The listing builds one solid part. Answer for the finished solid, in the listing's coordinates (mm). Face numbers are marked on the shaded views. Give positions to 0.01 mm unless a question says otherwise; leave off trailing zeros. Write each loop counter-clockwise with the first axis right and the second up, starting at its lowest first coordinate (ties: lowest second). Pieces come first, ordered by that corner, then holes. Notation, with made-up numbers: (-19.5, -1.5) - (34.5, -1.5) arc R25 cw to (34.5, 15.5) - close; hole circle Ø8 at (58.25, -21). An arc over 180 degrees is marked (long way). Use a Markdown table: item, result. Add a question column.
Autodesk Inventor part; units mm, degrees
ref_plane "YZ Plane" through (0, 0, 0) normal (1, 0, 0) x (0, 1, 0)
ref_plane "XZ Plane" through (0, 0, 0) normal (0, 1, 0) x (-1, 0, 0)
ref_plane "XY Plane" through (0, 0, 0) normal (0, 0, 1) x (1, 0, 0)
sketch "Sketch1" plane through (0, 0, 0) normal (0, 1, 0) x (-1, 0, 0)
  line L0 (-4, -15) -> (4, -15)
  line L1 (4, -15) -> (4, 15)
  line L2 (4, 15) -> (-4, 15)
  line L3 (-4, 15) -> (-4, -15)
  line L4 (-4, -15) -> (4, 15) construction
  line L5 (4, -15) -> (-4, 15) construction
  circle A0 centre (0, 0) radius 1.75
  dimension "d0" = 8
  dimension "d1" = 30
  dimension "d2" = 3.5
extrude "Extrusion1" add sketch "Sketch1" along normal blind 5
sketch "Sketch2" plane through (0, 5, 0) normal (0, 1, 0) x (1, 0, 0)
  circle A0 centre (0, 0) radius 1.75
  circle A1 centre (0, 0) radius 2.75 construction
  line L0 (-2.75, 1.5877) -> (0, 3.1754)
  line L1 (0, 3.1754) -> (2.75, 1.5877)
  line L2 (2.75, 1.5877) -> (2.75, -1.5877)
  line L3 (2.75, -1.5877) -> (0, -3.1754)
  line L4 (0, -3.1754) -> (-2.75, -1.5877)
  line L5 (-2.75, -1.5877) -> (-2.75, 1.5877)
  point P0 (-2.75, 0)
  dimension "d5" = 5.5
extrude "Extrusion2" cut sketch "Sketch2" against normal blind 2.4 contours A0 | L0 L1 L2 L3 L4 L5
sketch "Sketch3" plane through (0, 5, 0) normal (0, 1, 0) x (1, 0, 0)
  line L0 (-4, -15) -> (4, -15)
  line L1 (0, -15) -> (0, 15) construction
  line L2 (4, 15) -> (-4, 15)
  point P0 (0, 0)
  point P1 (0, -10)
  point P2 (0, 10)
  dimension "d8" = 5
  dimension "d9" = 5
hole "Hole1" at (0, 5, 10) at (0, 5, -10) direction (0, -1, 0) diameter 3.4 end through all
properties part number "turning clip bottom"
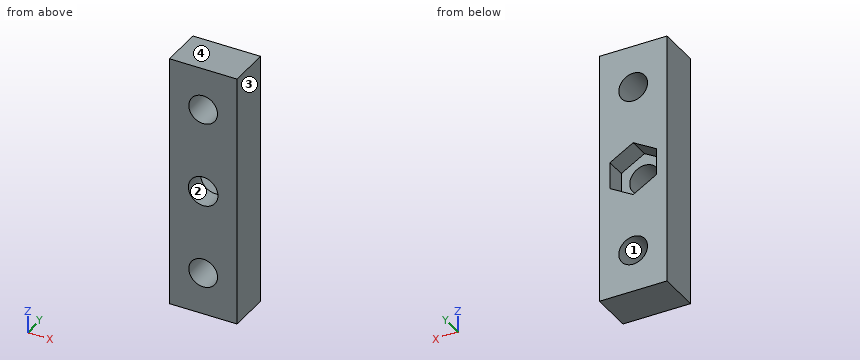
1. Consider L1, parallel to Z at x = 0, y = 1.35; L2, parallel to X at y = 1.7, z = 0; L3, parallel to Z at x = -0.75, y = 0.3. Determine where each line is inside the solid, lowest interval first. Write a range as [from, to].
2. The part is cut by section C-C (x = 0.75). Give the vertices of the cut face in (y, z).
3. Given P1, Ø4.5, axis at x = -0.5, z = 1, coming from the +Y side, flat-ended and moving along its own axis, determine where the tip first touches the part or whether it passes through.
4. The part is cut by section D-D (z = 0). Give the vertices of the cut face in (x, y).
5. The part is cut by section A-A (z = 10). Give the vertices of the cut face in (x, y), and give its area (3 significant figures).
6. The part is cut by section B-B (y = 4.05). Give the vertices of the cut face in (x, z).
7. For a pull along X with two mould halves and no side action, classify the marked faces 1, 2, 3 and 4 as released by +X, released by -X, zero draft, split by the parting line, or undercut.
Check values:
| question | item | result |
|---|---|---|
| 1 | L1 | z = [-15, -11.7], [-8.3, -1.75], [1.75, 8.3], [11.7, 15] |
| 1 | L2 | x = [-4, -1.75], [1.75, 4] |
| 1 | L3 | z = [-15, -11.53], [-8.47, -1.58], [1.58, 8.47], [11.53, 15] |
| 2 | outline | (0, -15) - (5, -15) - (5, -11.53) - (0, -11.53) - close; (0, -8.47) - (5, -8.47) - (5, -2.74) - (2.6, -2.74) - (2.6, -1.58) - (0, -1.58) - close; (0, 1.58) - (2.6, 1.58) - (2.6, 2.74) - (5, 2.74) - (5, 8.47) - (0, 8.47) - close; (0, 11.53) - (5, 11.53) - (5, 15) - (0, 15) - close |
| 3 | P1 | stops at y = 5 |
| 4 | outline | (-4, 0) - (-1.75, 0) - (-1.75, 2.6) - (-2.75, 2.6) - (-2.75, 5) - (-4, 5) - close; (1.75, 0) - (4, 0) - (4, 5) - (2.75, 5) - (2.75, 2.6) - (1.75, 2.6) - close |
| 5 | outline | (-4, 0) - (-1.7, 0) - (-1.7, 5) - (-4, 5) - close; (1.7, 0) - (4, 0) - (4, 5) - (1.7, 5) - close |
| 5 | area | 23.0 mm2 |
| 6 | outline | (-4, -15) - (4, -15) - (4, 15) - (-4, 15) - close; hole (-2.75, -1.59) - (0, -3.18) - (2.75, -1.59) - (2.75, 1.59) - (0, 3.18) - (-2.75, 1.59) - close; hole circle Ø3.4 at (0, -10); hole circle Ø3.4 at (0, 10) |
| 7 | face 1 | undercut |
| 7 | face 2 | undercut |
| 7 | face 3 | released by +X |
| 7 | face 4 | zero draft |
